from build123d import *

# Parameters (mm, degrees)
CUT_EXTRUDE1_DEPTH      = 20
SKETCH6_R               = 8
CUT_EXTRUDE2_DEPTH      = 30
SKETCH7_R               = 3
CUT_EXTRUDE3_DEPTH      = 30
CUT_EXTRUDE3_DEPTH_BACK = 30


with BuildPart() as part:
    # Sketch2 → Revolve1 (revolve)
    with BuildSketch(Plane(origin=(0, 0, 0), x_dir=(0, 0, -1), z_dir=(1, 0, 0))):
        Polygon((0, 13), (0, 0), (40, 0), (40, 3), (25, 3), (25, 13), align=None)
    revolve(axis=Axis((0, 13, -25), (0, 0, 1)))

    # Sketch5 → Cut-Extrude1 (cut)
    with BuildSketch(Plane.XY):
        with BuildLine():
            ThreePointArc((13, 13), (11.708749973, 18.648466524), (8.091511681, 23.174843424))
            Line((8.091511681, 23.174843424), (8.091511681, 2.825156576))
            ThreePointArc((8.091511681, 2.825156576), (11.708749973, 7.351533476), (13, 13))
        make_face()
        with BuildLine():
            Line((-8.091511681, 2.825156576), (-8.091511681, 23.174843424))
            ThreePointArc((-8.091511681, 23.174843424), (-13, 13), (-8.091511681, 2.825156576))
        make_face()
    extrude(amount=-CUT_EXTRUDE1_DEPTH, mode=Mode.SUBTRACT)

    # Sketch6 → Cut-Extrude2 (cut)
    with BuildSketch(Plane(origin=(8.091511681, 0, 0), x_dir=(0, 0, -1), z_dir=(1, 0, 0))):
        with Locations((10, 13)):
            Circle(SKETCH6_R)
    extrude(amount=-CUT_EXTRUDE2_DEPTH, mode=Mode.SUBTRACT)

    # Sketch7 → Cut-Extrude3 (cut, two sides)
    with BuildSketch(Plane(origin=(0, 0, 0), x_dir=(0, 0, -1), z_dir=(1, 0, 0))) as cut_extrude3_sk:
        with Locations((36, 13)):
            Circle(SKETCH7_R)
    extrude(amount=CUT_EXTRUDE3_DEPTH, mode=Mode.SUBTRACT)
    extrude(cut_extrude3_sk.sketch, amount=-CUT_EXTRUDE3_DEPTH_BACK, mode=Mode.SUBTRACT)


solid = part.part
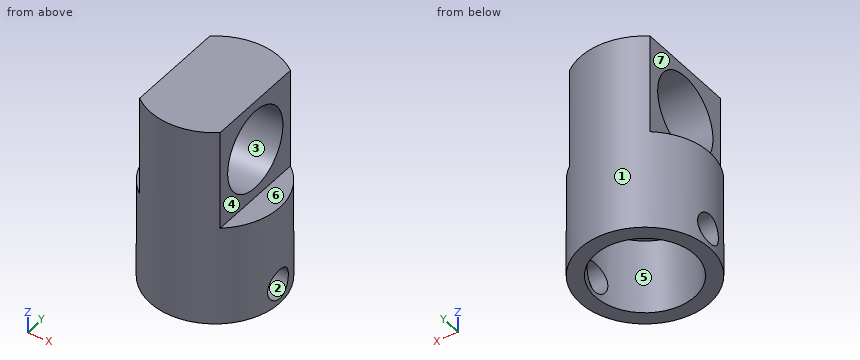
Geometry check sheet. Reference: the model listing, model coordinates, mm. Face numbers are marked on the shaded views. A direction names the side the tool comes from. Round coordinates to 2 decimals unless told otherwise and drop trailing zeros. Write each loop counter-clockwise with the first axis right and the second up, starting at its lowest first coordinate (ties: lowest second). Pieces come first, ordered by that corner, then holes. Notation, with made-up numbers: (52, 73) -> (105, 73) arc R24 ccw to (105, 90) -> close; hole circle Ø10 at (-15, 81). An arc over 180 degrees is marked (long way). One line per item, written item: value. Start each with the question number.
(1) Cross-section at D-D, the plane z = -36. Record the cut outline in (x, y), and give its area (3 significant figures).
(2) Cross-section at C-C, the plane y = 5.75. Record the cut outline in (x, z).
(3) Cross-section at A-A, the plane z = -10. Record the cut outline in (x, y).
(4) Scan lines: line 1 (X direction, y = 13, z = -29.5); line 2 (Z direction, x = 10.2, y = 13); line 3 (X direction, y = 22.25, z = -8.5). Record each from-to range of solid material in increasing order. Write a range as [from, to].
(5) Cross-section at B-B, the plane x = 0. Record the cut outline in (y, z), and give its area (3 significant figures).
(6) Access from +Z, -Z, +X, -X, +Y, -Y to the whole of each face (thin tool, end or side, straight path). Record for the marked faces 5, 6 and 7.
(7) Draft check along Y on the marked faces 1, 2, 3 and 4. Enter one of: +Y half, -Y half, draft (parallel to the pull), parting line (faces both ways), or undercut.
(8) Go/stop test with flat-tipped pins: pin 1 Ø8 at (x, y) = (-1.5, 14) entering from -Z; pin 2 Ø6 at (x, z) = (-8, -27.5) entering from +Y; pin 3 Ø1 at (x, z) = (2, -26) entering from +Y. Record where each tip stops, or that it passes through.
Answer:
1. outline: (-12.65, 10) arc R13 ccw to (12.65, 10) -> (9.54, 10) arc R10 cw to (-9.54, 10) -> close; (-12.65, 16) -> (-9.54, 16) arc R10 cw to (9.54, 16) -> (12.65, 16) arc R13 ccw to start
1. area: 180 mm²
2. outline: (-10.79, -40) -> (-6.89, -40) -> (-6.89, -25) -> (6.89, -25) -> (6.89, -40) -> (10.79, -40) -> (10.79, -20) -> (8.09, -20) -> (8.09, -13.38) -> (-8.09, -13.38) -> (-8.09, -20) -> (-10.79, -20) -> close; (-8.09, -6.62) -> (8.09, -6.62) -> (8.09, 0) -> (-8.09, 0) -> close
3. outline: (-8.09, 2.83) arc R13 ccw to (8.09, 2.83) -> (8.09, 5) -> (-8.09, 5) -> close; (-8.09, 21) -> (8.09, 21) -> (8.09, 23.17) arc R13 ccw to (-8.09, 23.17) -> close
4. line 1: [-13, -10], [10, 13]
4. line 2: [-40, -39], [-33, -20]
4. line 3: [-8.09, 8.09]
5. outline: (0, -40) -> (3, -40) -> (3, -25) -> (23, -25) -> (23, -40) -> (26, -40) -> (26, 0) -> (0, 0) -> close; hole circle Ø16 at (13, -10)
5. area: 539 mm²
6. face 5: -Z
6. face 6: +Z, +X, +Y, -Y
6. face 7: +Z, -X, +Y, -Y
7. face 1: parting line
7. face 2: undercut
7. face 3: undercut
7. face 4: draft
8. pin 1: z = -25
8. pin 2: y = 25
8. pin 3: y = 25.91
